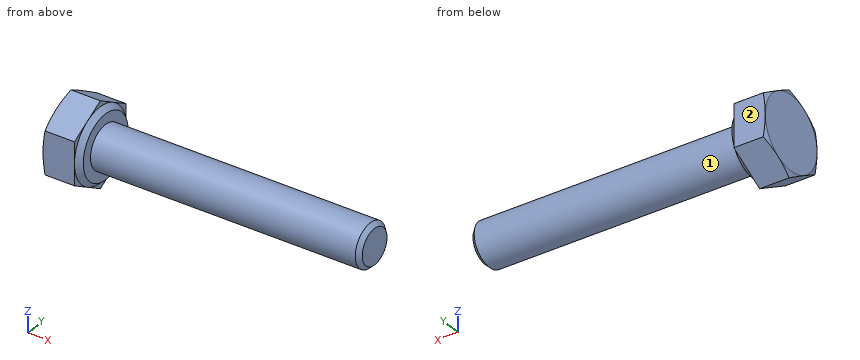
from build123d import *

# Parameters (mm, degrees)
BASEHEAD_DEPTH = 2.925
SKETCH3_R      = 2
BASEBODY_DEPTH = 25


with BuildPart() as part:
    # Sketch-BaseHead → BaseHead (new body)
    with BuildSketch(Plane(origin=(0, 0, 0), x_dir=(0, 0, -1), z_dir=(1, 0, 0))):
        Polygon((3.914434825, 0), (1.957217413, 3.39), (-1.957217413, 3.39), (-3.914434825, 0), (-1.957217413, -3.39), (1.957217413, -3.39), align=None)
    extrude(amount=BASEHEAD_DEPTH)

    # Sketch4 → HeadChamfer (revolve, cut)
    with BuildSketch(Plane(origin=(-0.264637255, 0, 5.916896391), x_dir=(0, 0, -1), z_dir=(0, 1, 0))):
        Polygon((9.831331216, -0.264637255), (9.306896391, -0.264637255), (9.831331216, -0.455515922), align=None)
    revolve(axis=Axis((-4.001564945, 0, 0), (1, 0, 0)), mode=Mode.SUBTRACT)

    # Sketch1 → Revolve1 (revolve)
    with BuildSketch(Plane.XY, mode=Mode.PRIVATE) as revolve1_sk:
        Polygon((2.925, 0), (3.425, 0), (3.425, -2.94), (2.925, -3.39), align=None)
    revolve(revolve1_sk.sketch.rotate(Axis((-4.001564945, 0, 0), (1, 0, 0)), 270), axis=Axis((-4.001564945, 0, 0), (1, 0, 0)))

    # Sketch3 → BaseBody (add)
    with BuildSketch(Plane(origin=(3.425, 0, 0), x_dir=(0, 0, -1), z_dir=(1, 0, 0))):
        Circle(SKETCH3_R)
    extrude(amount=BASEBODY_DEPTH)

    # Chamfer1: read off the stored shape, not the designer's step
    # Chamfer1 outline → Chamfer1 (revolve, cut)
    with BuildSketch(Plane.YX):
        Polygon((2, 28.425), (1.621, 28.425), (2, 28.046), align=None)
    revolve(axis=Axis((0, 0, 0), (1, 0, 0)), mode=Mode.SUBTRACT)


solid = part.part
Design review of the part built by this model. Coordinates are the model's own, in mm. Face numbers are marked on the shaded views. A direction names the side the tool comes from. Coordinates: 2 decimals unless noted, no trailing zeros. Order: outer loops, then holes, each group sorted by start corner. A loop starts at its lowest first (then second) coordinate and runs counter-clockwise, first axis right, second up. Notation, with made-up numbers: (28.5, -19.5) -> (69.5, -19.5) arc R35 cw to (69.5, 17.5) -> close; hole circle Ø3 at (4.5, 45.25). An arc over 180 degrees is marked (long way). Use one line per item in the form item = value. Start each with the question number.
(1) For the marked faces 1 and 2, list the 3-axis set-ups (+Z, -Z, +X, -X, +Y, -Y) from which the entire face can be reached by the end or side of a thin tool; tool diameter is ignored.
(2) Insertion check: pin 1 (0.5 mm diameter, centred on y = -0.5, z = -3.5, fed in from +X); pin 2 (1.1 mm diameter, centred on y = -0.5, z = 3.5, fed in from +X); pin 3 (1.5 mm diameter, centred on x = 9, z = 1.5, fed in from +Y). Each pin has a flat end and moves straight along its axis. Give the tip position at first contact, or say it passes through.
(3) For probe 1 along X at (y, z) = (2.25, 1) (3 decimals); probe 2 along Z at (x, y) = (23.75, 0); probe 3 along Y at (x, z) = (15.5, -1.75), list the stretches that pass through material, from the lowest coordinate up.
(4) Add section A-A on x = 11. State the section outline as (y, z) points.
Answer block:
q1.face_1 = +X
q1.face_2 = +Z, -Z, +X, -X, +Y
q2.pin_1 = 3.04
q2.pin_2 = 3.37
q2.pin_3 = 1.85
q3.probe_1 = 0 to 3.425
q3.probe_2 = -2 to 2
q3.probe_3 = -0.97 to 0.97
q4.outline = circle Ø4 at (0, 0)
